```python
from build123d import *

# Parameters (mm, degrees)
CROQUIS1_R              = 1.75
CROQUIS1_R_2            = 11.25
CROQUIS1_R_3            = 2.65
CROQUIS1_R_4            = 2.5
SALIENTE_EXTRUIR1_DEPTH = 6
CORTAR_EXTRUIR1_DEPTH   = 194.095831131


with BuildPart() as part:
    # Croquis1 → Saliente-Extruir1 (new body)
    with BuildSketch(Plane(origin=(0, 0, 0), x_dir=(1, 0, 0), z_dir=(0, 1, 0))):
        Polygon((-155, -65), (-43.397871348, -65), (-35, -65), (-35, -71), (-35, -109), (-35, -115), (-29, -115), (29, -115), (35, -115), (35, -109), (35, -71), (35, -65), (51, -65), (155, -65), (155, 65), (51, 65), (35, 65), (35, 71), (35, 107), (35, 113), (29, 113), (-29, 113), (-35, 113), (-35, 107), (-35, 71), (-35, 65), (-43.397871348, 65), (-155, 65), align=None)
        with Locations(Location((-146.655, 15.495, 0), (0, 0, 270))):
            Circle(CROQUIS1_R, mode=Mode.SUBTRACT)
        with Locations(Location((-115.665, 15.495, 0), (0, 0, 270))):
            Circle(CROQUIS1_R, mode=Mode.SUBTRACT)
        with Locations(Location((-115.665, -15.495, 0), (0, 0, 270))):
            Circle(CROQUIS1_R, mode=Mode.SUBTRACT)
        with Locations(Location((-146.655, -15.495, 0), (0, 0, 270))):
            Circle(CROQUIS1_R, mode=Mode.SUBTRACT)
        with Locations(Location((-131.16, 0, 0), (0, 0, 270))):
            Circle(CROQUIS1_R_2, mode=Mode.SUBTRACT)
        with Locations(Location((135, 0, 0), (0, 0, 270))):
            Circle(CROQUIS1_R_3, mode=Mode.SUBTRACT)
        with Locations(Location((-148, -60, 0), (0, 0, 270))):
            Circle(CROQUIS1_R_4, mode=Mode.SUBTRACT)
        with Locations(Location((-148, -28, 0), (0, 0, 270))):
            Circle(CROQUIS1_R_4, mode=Mode.SUBTRACT)
        with Locations(Location((148, -60, 0), (0, 0, 270))):
            Circle(CROQUIS1_R_4, mode=Mode.SUBTRACT)
        with Locations(Location((148, -28, 0), (0, 0, 270))):
            Circle(CROQUIS1_R_4, mode=Mode.SUBTRACT)
        with Locations(Location((148, 60, 0), (0, 0, 90))):
            Circle(CROQUIS1_R_4, mode=Mode.SUBTRACT)
        with Locations(Location((148, 28, 0), (0, 0, 90))):
            Circle(CROQUIS1_R_4, mode=Mode.SUBTRACT)
        with Locations(Location((-148, 60, 0), (0, 0, 90))):
            Circle(CROQUIS1_R_4, mode=Mode.SUBTRACT)
        with Locations(Location((-148, 28, 0), (0, 0, 90))):
            Circle(CROQUIS1_R_4, mode=Mode.SUBTRACT)
        with Locations(Location((-27, 99, 0), (0, 0, 270))):
            Circle(CROQUIS1_R_4, mode=Mode.SUBTRACT)
        with Locations(Location((-27, 77, 0), (0, 0, 270))):
            Circle(CROQUIS1_R_4, mode=Mode.SUBTRACT)
        with Locations(Location((27, 77, 0), (0, 0, 90))):
            Circle(CROQUIS1_R_4, mode=Mode.SUBTRACT)
        with Locations(Location((27, 99, 0), (0, 0, 90))):
            Circle(CROQUIS1_R_4, mode=Mode.SUBTRACT)
        with Locations(Location((27, -101, 0), (0, 0, 270))):
            Circle(CROQUIS1_R_4, mode=Mode.SUBTRACT)
        with Locations(Location((27, -79, 0), (0, 0, 270))):
            Circle(CROQUIS1_R_4, mode=Mode.SUBTRACT)
        with Locations(Location((-27, -101, 0), (0, 0, 90))):
            Circle(CROQUIS1_R_4, mode=Mode.SUBTRACT)
        with Locations(Location((-27, -79, 0), (0, 0, 90))):
            Circle(CROQUIS1_R_4, mode=Mode.SUBTRACT)
    extrude(amount=SALIENTE_EXTRUIR1_DEPTH)

    # Croquis3 → Cortar-Extruir1 (cut, through all)
    with BuildSketch(Plane(origin=(0, 6, 0), x_dir=(1, 0, 0), z_dir=(0, 1, 0))):
        with BuildLine():
            Line((136, 35), (121, 35))
            ThreePointArc((121, 35), (118.9, 37.1), (121, 39.2))
            Line((121, 39.2), (136, 39.2))
            ThreePointArc((136, 39.2), (138.1, 37.1), (136, 35))
        make_face()
        with BuildLine():
            Line((136, 21.2), (121, 21.2))
            ThreePointArc((121, 21.2), (118.9, 19.1), (121, 17))
            Line((121, 17), (136, 17))
            ThreePointArc((136, 17), (138.1, 19.1), (136, 21.2))
        make_face()
    extrude(amount=-CORTAR_EXTRUIR1_DEPTH, mode=Mode.SUBTRACT)


solid = part.part
```
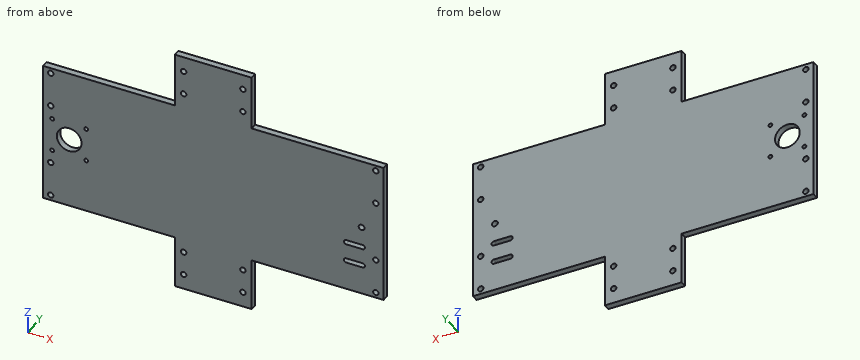
Geometry: final body of the model. Coordinates: model frame, mm. Coordinates: 2 decimals unless noted, no trailing zeros. Write each loop counter-clockwise with the first axis right and the second up, starting at its lowest first coordinate (ties: lowest second). Pieces come first, ordered by that corner, then holes. Notation, with made-up numbers: M 51.25,-25 L 55.25,-25 A12 cw 55.25,-21 Z; hole C 29,-31 d8. An arc over 180 degrees is marked long. Answer as CSV lines item,"result". Start each with the question number.
Q1. Cut plane B-B on z = 7.5. Return the cut outline in (x, y).
Q2. Cut plane D-D on y = 3.2. Count the separate pieces of the cut face and the enclosed holes in it, then the cut area to 3 significant figures.
Q3. Pin query (flat end, axial travel): P1, Ø1.5, axis at x = 48, y = 3.5, coming from the -Z side. Return the tip coordinate at first contact, or that it passes through.
Q4. Cut plane A-A on x = -131.16. Return the cut outline in (y, z).
Q5. Line query: line 1 (X direction, y = 5.2, z = 101); line 2 (X direction, y = 4.25, z = -28); line 3 (Z direction, x = 130, y = 1.3). Output: solid intervals per line, ascending. Write a range as from..to.
Q6. Cut plane C-C on z = -84. Return the cut outline in (x, y), then the cut area to 3 significant figures.
Findings below:
1,outline,"M -155,0 L -139.55,0 L -139.55,6 L -155,6 Z; M -122.77,0 L 155,0 L 155,6 L -122.77,6 Z"
2,separate pieces,"1"
2,enclosed holes,"24"
2,area,"46,200 mm2"
3,P1,"stops at z = -65"
4,outline,"M 0,-65 L 6,-65 L 6,-11.25 L 0,-11.25 Z; M 0,11.25 L 6,11.25 L 6,65 L 0,65 Z"
5,line 1,"x = -35..-29.5, -24.5..24.5, 29.5..35"
5,line 2,"x = -155..-150.5, -145.5..145.5, 150.5..155"
5,line 3,"z = -65..-39.2, -35..-21.2, -17..65"
6,outline,"M -35,0 L 35,0 L 35,6 L -35,6 Z"
6,area,"420 mm2"
